Can you work these out from the model? Positions are in its coordinate system, mm. A direction names the side the tool comes from. Coordinates: 2 decimals unless noted, no trailing zeros. Write each loop counter-clockwise with the first axis right and the second up, starting at its lowest first coordinate (ties: lowest second). Pieces come first, ordered by that corner, then holes. Notation, with made-up numbers: M -10.5,18 L -1.5,18 A28 ccw -1.5,42 Z; hole C 46,-23 d10. An arc over 180 degrees is marked long. Use one line per item in the form item = value. Start each with the question number.
```python
from build123d import *

# Parameters (mm, degrees)
ESQUISSE1_W             = 21
ESQUISSE1_H             = 13
BOSS_EXTRU_1_DEPTH      = 2
ESQUISSE2_R             = 1.25
ENL_V_MAT_EXTRU_1_DEPTH = 2
BOSS_EXTRU_2_DEPTH      = 9
BOSS_EXTRU_2_DEPTH_BACK = 4
ESQUISSE3_W             = 2.5
ESQUISSE3_H             = 13


with BuildPart() as part:
    # Esquisse1 → Boss.-Extru.1 (new body)
    with BuildSketch(Plane.XY):
        with Locations((10.5, 6.5)):
            Rectangle(ESQUISSE1_W, ESQUISSE1_H)
    extrude(amount=BOSS_EXTRU_1_DEPTH)

    # Esquisse2 → Enlèv. mat.-Extru.1 (cut)
    with BuildSketch(Plane.XY.offset(2)):
        with Locations((2.5, 2.5)):
            Circle(ESQUISSE2_R)
    extrude(amount=-ENL_V_MAT_EXTRU_1_DEPTH, mode=Mode.SUBTRACT)

    # Esquisse3 → Boss.-Extru.2 (add, two sides: drawn at the far end of the back side and taken through both)
    with BuildSketch(Plane.XY.offset(2).offset(-BOSS_EXTRU_2_DEPTH_BACK)):
        with Locations((19.75, 6.5)):
            Rectangle(ESQUISSE3_W, ESQUISSE3_H)
    extrude(amount=BOSS_EXTRU_2_DEPTH + BOSS_EXTRU_2_DEPTH_BACK)


solid = part.part
```
1) Suppose I cut it at B-B on x = 3.5. Please give me the cut outline in (y, z), and give its area (3 significant figures).
2) Please list where these lines run through material, in increasing order: line 1 (Y direction, x = 2.5, z = 1.4); line 2 (Z direction, x = 6.5, y = 11); line 3 (X direction, y = 7.25, z = 7.5).
3) If we mould it in two halves opening along Y, with no side actions, what happens to faces 4 (the face through (18.5, 6, 6)), 5 (the face through (3.69, 2.88, 1.01)), 6 (the face through (14, 0, 1))? For each: +Y half, -Y half, draft (parallel to the pull), parting line (faces both ways), or undercut.
4) Will these pins go through, and if not, where does the flat tip stop? pin 1 Ø2 at (x, y) = (2.5, 6.5) entering from +Z; pin 2 Ø4 at (x, z) = (15.5, 9) entering from -Y; pin 3 Ø6.5 at (x, y) = (6, 5) entering from -Z; pin 4 Ø1 at (y, z) = (3.5, 4.5) entering from -X.
5) Suppose I cut it at D-D on z = 0.25. Please give me the cut outline in (x, y), and give its area (3 significant figures).
6) Which directions (+Z, -Z, +X, -X, +Y, -Y) give clear straight access to the entire face, cutting with the end or side of a thin tool? Please do faces 1 (the face through (9, 7, 2)), 2 (the face through (21, 6, 4)), 3 (the face through (18.5, 6, -1)).
7) Suppose I cut it at A-A on y = 1.5. Please give me the cut outline in (x, z), and give its area (3 significant figures).
8) Suppose I cut it at C-C on y = 8.5. Please give me the cut outline in (x, z).
Computed values:
q1.outline = M 0,0 L 1.75,0 L 1.75,2 L 0,2 Z; M 3.25,0 L 13,0 L 13,2 L 3.25,2 Z
q1.area = 23.0 mm²
q2.line_1 = 0 to 1.25, 3.75 to 13
q2.line_2 = 0 to 2
q2.line_3 = 18.5 to 21
q3.face_4 = draft
q3.face_5 = undercut
q3.face_6 = -Y half
q4.pin_1 = 2
q4.pin_2 = through
q4.pin_3 = 0
q4.pin_4 = 18.5
q5.outline = M 0,0 L 21,0 L 21,13 L 0,13 Z; hole C 2.5,2.5 d2.5
q5.area = 268 mm²
q6.face_1 = +Z, -X, +Y, -Y
q6.face_2 = +Z, -Z, +X, +Y, -Y
q6.face_3 = -Z, -X, +Y, -Y
q7.outline = M 0,0 L 1.75,0 L 1.75,2 L 0,2 Z; M 3.25,0 L 18.5,0 L 18.5,-2 L 21,-2 L 21,11 L 18.5,11 L 18.5,2 L 3.25,2 Z
q7.area = 66.5 mm²
q8.outline = M 0,0 L 18.5,0 L 18.5,-2 L 21,-2 L 21,11 L 18.5,11 L 18.5,2 L 0,2 Z
